```python
from build123d import *

# Parameters (mm, degrees)
F0_R     = 11
F0_R_2   = 9.5
F1_DEPTH = 4
F2_R     = 5.5
F2_R_2   = 4
F3_DEPTH = 4
F4_R     = 9.5
F4_R_2   = 5.5
F5_DEPTH = 3.25


with BuildPart() as f1:
    # F0 (on Front) → F1 (new body, symmetric)
    with BuildSketch(Plane.XZ):
        Circle(F0_R)
        Circle(F0_R_2, mode=Mode.SUBTRACT)
    extrude(amount=F1_DEPTH, both=True)



with BuildPart() as f3:
    # F2 (on Front) → F3 (new body, symmetric)
    with BuildSketch(Plane.XZ):
        Circle(F2_R)
        Circle(F2_R_2, mode=Mode.SUBTRACT)
    extrude(amount=F3_DEPTH, both=True)


with BuildPart() as f1_1:
    add(f1.part)

    add(f3.part)  # F5 merges F3
    # F4 (on Front) → F5 (join, symmetric)
    with BuildSketch(Plane.XZ):
        Circle(F4_R)
        Circle(F4_R_2, mode=Mode.SUBTRACT)
    extrude(amount=F5_DEPTH, both=True)


solid = f1_1.part
```
Here's how the part is built. I have some questions about the finished solid (model axes, mm). A direction names the side the tool comes from. Give positions to 0.01 mm unless a question says otherwise; leave off trailing zeros. Write each loop counter-clockwise with the first axis right and the second up, starting at its lowest first coordinate (ties: lowest second). Pieces come first, ordered by that corner, then holes.
(1) On a 3-axis mill with a long thin cutter (end or side, diameter ignored), from which of +Z, -Z, +X, -X, +Y, -Y can I reach the whole of each face in a straight line? I mean faces 4 (the face through (-4, -4, -2)), 5 (the face through (4, 3.25, -4)), 6 (the face through (4, -3.25, -4)). Say none if no direction works.
Output values:
face 4: +Z, -Z, +X, -X, -Y
face 5: +Y
face 6: -Y
(2) Thinking about a two-plate mould opening in X: for faces 1 (the face through (-10, -4, 0)), 2 (the face through (-2.38, -0.06, -10.74)), 3 (the face through (-1.19, 3.62, -5.37)), which applies, pulls with the +X half, pulls with the -X half, needs draft (parallel to the pull), parting line crosses it, or undercut?
Output values:
face 1: needs draft
face 2: parting line crosses it
face 3: undercut
(3) Imagine slicing it at D-D, the plane x = 8.5. Write out the boundary of the cut face in (y, z).
Output values:
outline: (-4, -6.98) - (4, -6.98) - (4, -4.24) - (3.25, -4.24) - (3.25, 4.24) - (4, 4.24) - (4, 6.98) - (-4, 6.98) - (-4, 4.24) - (-3.25, 4.24) - (-3.25, -4.24) - (-4, -4.24) - close
(4) If I drill on L1, parallel to Z at x = 0, y = 3.8; L2, parallel to Z at x = 0, y = -1.75; L3, parallel to Y at x = 9.25, z = 1.75, over which ranges is the centre line in solid material (lowest first)?
Output values:
L1: z = -11 to -9.5, -5.5 to -4, 4 to 5.5, 9.5 to 11
L2: z = -11 to -4, 4 to 11
L3: y = -3.25 to 3.25
(5) Will these pins go through, and if not, where does the flat tip stop? pin 1 (6.5 mm diameter, centred on x = 0, z = 0, fed in from -Y); pin 2 (1.5 mm diameter, centred on y = 3, z = -1, fed in from -X); pin 3 (5.5 mm diameter, centred on x = 0, z = 2, fed in from +Y); pin 4 (4 mm diameter, centred on x = -8.5, y = -1, fed in from +Z).
Output values:
pin 1: passes through
pin 2: stops at x = -11
pin 3: stops at y = 4
pin 4: stops at z = 8.87
(6) Imagine slicing it at B-B, the plane x = 0. Write out the boundary of the cut face in (y, z), and give its area (4 significant figures).
Output values:
outline: (-4, -11) - (4, -11) - (4, -9.5) - (3.25, -9.5) - (3.25, -5.5) - (4, -5.5) - (4, -4) - (-4, -4) - (-4, -5.5) - (-3.25, -5.5) - (-3.25, -9.5) - (-4, -9.5) - close; (-4, 4) - (4, 4) - (4, 5.5) - (3.25, 5.5) - (3.25, 9.5) - (4, 9.5) - (4, 11) - (-4, 11) - (-4, 9.5) - (-3.25, 9.5) - (-3.25, 5.5) - (-4, 5.5) - close
area: 100.0 mm2
(7) Imagine slicing it at C-C, the plane y = 0. Write out the boundary of the cut face in (x, z), and give its area (3 significant figures).
Output values:
outline: circle Ø22 at (0, 0); hole circle Ø8 at (0, 0)
area: 330 mm2
(8) Imagine slicing it at A-A, the plane z = 0. Write out the boundary of the cut face in (x, y), and give its area (4 significant figures).
Output values:
outline: (-11, -4) - (-9.5, -4) - (-9.5, -3.25) - (-5.5, -3.25) - (-5.5, -4) - (-4, -4) - (-4, 4) - (-5.5, 4) - (-5.5, 3.25) - (-9.5, 3.25) - (-9.5, 4) - (-11, 4) - close; (4, -4) - (5.5, -4) - (5.5, -3.25) - (9.5, -3.25) - (9.5, -4) - (11, -4) - (11, 4) - (9.5, 4) - (9.5, 3.25) - (5.5, 3.25) - (5.5, 4) - (4, 4) - close
area: 100.0 mm2
